The model under review builds one solid part; all positions refer to its coordinate system, in mm. A direction names the side the tool comes from. Coordinates: 2 decimals unless noted, no trailing zeros. Order: outer loops, then holes, each group sorted by start corner. A loop starts at its lowest first (then second) coordinate and runs counter-clockwise, first axis right, second up. Notation, with made-up numbers: (26.5, 46) -> (47.5, 46) arc R31 cw to (47.5, 72) -> close; hole circle Ø1 at (-31.5, 41). An arc over 180 degrees is marked (long way). Use one line per item in the form item = value.
from build123d import *

# Parameters (mm, degrees)
SKETCH_1_W           = 100
SKETCH_1_H           = 125
EXTRUDE_1_DEPTH      = 3
SKETCH_2_W           = 5
SKETCH_2_H           = 100
EXTRUDE_2_DEPTH      = 75
SKETCH_3_R           = 2.25
CUT_EXTRUDE_1_DEPTH  = 85
SKETCH_4_W           = 40
SKETCH_4_H           = 41.42
CUT_EXTRUDE_2_DEPTH  = 85
CHAMFER_1_SIZE       = 10
SKETCH_5_W           = 10
SKETCH_5_H           = 30
CUT_EXTRUDE_3_DEPTH  = 85
SKETCH_11_R          = 1.7
CUT_EXTRUDE_5_DEPTH  = 10
SKETCH_12_R          = 1.7
CUT_EXTRUDE_6_DEPTH  = 25
SKETCH_13_R          = 2.3
SKETCH_13_R_2        = 15
CUT_EXTRUDE_9_DEPTH  = 105
SKETCH_14_W          = 15
SKETCH_14_H          = 41.42
CUT_EXTRUDE_10_DEPTH = 83
SKETCH_15_W          = 38.97610678
SKETCH_15_H          = 41.42
CUT_EXTRUDE_11_DEPTH = 83
SKETCH_16_R          = 1.7
CUT_EXTRUDE_12_DEPTH = 83
SKETCH_17_R          = 2.15
CUT_EXTRUDE_13_DEPTH = 83
CHAMFER_2_SIZE       = 8


with BuildPart() as part:
    # 草图1 → 凸台-拉伸1 (new body)
    with BuildSketch(Plane(origin=(0, 0, 0), x_dir=(1, 0, 0), z_dir=(0, 1, 0))):
        Rectangle(SKETCH_1_W, SKETCH_1_H)
    extrude(amount=EXTRUDE_1_DEPTH)

    # 草图2 → 凸台-拉伸2 (add)
    with BuildSketch(Plane.XZ):
        with Locations((-34.5, 0)):
            Rectangle(SKETCH_2_W, SKETCH_2_H)
        with Locations((34.5, 0)):
            Rectangle(SKETCH_2_W, SKETCH_2_H)
    extrude(amount=EXTRUDE_2_DEPTH)

    # 草图3 → 切除-拉伸1 (cut)
    with BuildSketch(Plane.ZY.offset(37)):
        with Locations((-4.925, -12)):
            Circle(SKETCH_3_R)
        with Locations((4.925, -12)):
            Circle(SKETCH_3_R)
        with Locations((-4.925, -61.42)):
            Circle(SKETCH_3_R)
        with Locations((4.925, -61.42)):
            Circle(SKETCH_3_R)
        with Locations((14.775, -12)):
            Circle(SKETCH_3_R)
        with Locations((14.775, -61.42)):
            Circle(SKETCH_3_R)
        with Locations((-14.775, -61.42)):
            Circle(SKETCH_3_R)
        with Locations((-14.775, -12)):
            Circle(SKETCH_3_R)
    extrude(amount=-CUT_EXTRUDE_1_DEPTH, mode=Mode.SUBTRACT)

    # 草图4 → 切除-拉伸2 (cut)
    with BuildSketch(Plane.ZY.offset(37)):
        with Locations((0, -36.71)):
            Rectangle(SKETCH_4_W, SKETCH_4_H)
    extrude(amount=-CUT_EXTRUDE_2_DEPTH, mode=Mode.SUBTRACT)

    # 倒角1
    chamfer_1_edges = [part.edges().sort_by_distance(p)[0] for p in [
        (-34.5, -75, 50),
        (-34.5, -75, -50),
        (34.5, -75, 50),
        (34.5, -75, -50),
    ]]
    chamfer(chamfer_1_edges, length=CHAMFER_1_SIZE)

    # 草图5 → 切除-拉伸3 (cut)
    with BuildSketch(Plane(origin=(0, 3, 0), x_dir=(1, 0, 0), z_dir=(0, 1, 0))):
        with Locations((-25, 0)):
            Rectangle(SKETCH_5_W, SKETCH_5_H)
        with Locations((25, 0)):
            Rectangle(SKETCH_5_W, SKETCH_5_H)
    extrude(amount=-CUT_EXTRUDE_3_DEPTH, mode=Mode.SUBTRACT)

    # 草图11 → 切除-拉伸5 (cut)
    with BuildSketch(Plane.XZ):
        with Locations(Location((-44, 50.5, 0), (0, 0, 270))):
            Circle(SKETCH_11_R)
        with Locations(Location((-44, 38.5, 0), (0, 0, 270))):
            Circle(SKETCH_11_R)
        with Locations(Location((-44, 26.5, 0), (0, 0, 270))):
            Circle(SKETCH_11_R)
        with Locations(Location((44, 26.5, 0), (0, 0, 270))):
            Circle(SKETCH_11_R)
        with Locations(Location((44, 38.5, 0), (0, 0, 270))):
            Circle(SKETCH_11_R)
        with Locations(Location((44, 50.5, 0), (0, 0, 270))):
            Circle(SKETCH_11_R)
        with Locations(Location((44, -50.5, 0), (0, 0, 270))):
            Circle(SKETCH_11_R)
        with Locations(Location((44, -38.5, 0), (0, 0, 270))):
            Circle(SKETCH_11_R)
        with Locations(Location((44, -26.5, 0), (0, 0, 270))):
            Circle(SKETCH_11_R)
        with Locations(Location((-44, -26.5, 0), (0, 0, 270))):
            Circle(SKETCH_11_R)
        with Locations(Location((-44, -38.5, 0), (0, 0, 270))):
            Circle(SKETCH_11_R)
        with Locations(Location((-44, -50.5, 0), (0, 0, 270))):
            Circle(SKETCH_11_R)
    extrude(amount=-CUT_EXTRUDE_5_DEPTH, mode=Mode.SUBTRACT)

    # 草图12 → 切除-拉伸6 (cut)
    with BuildSketch(Plane(origin=(0, 3, 0), x_dir=(1, 0, 0), z_dir=(0, 1, 0))):
        with Locations(Location((-27.75, 54.5, 0), (0, 0, 270))):
            Circle(SKETCH_12_R)
        with Locations(Location((-27.75, 35.7, 0), (0, 0, 270))):
            Circle(SKETCH_12_R)
        with Locations(Location((27.75, 35.7, 0), (0, 0, 90))):
            Circle(SKETCH_12_R)
        with Locations(Location((27.75, 54.5, 0), (0, 0, 90))):
            Circle(SKETCH_12_R)
        with Locations(Location((27.75, -54.5, 0), (0, 0, 270))):
            Circle(SKETCH_12_R)
        with Locations(Location((27.75, -35.7, 0), (0, 0, 270))):
            Circle(SKETCH_12_R)
        with Locations(Location((-27.75, -35.7, 0), (0, 0, 90))):
            Circle(SKETCH_12_R)
        with Locations(Location((-27.75, -54.5, 0), (0, 0, 90))):
            Circle(SKETCH_12_R)
    extrude(amount=-CUT_EXTRUDE_6_DEPTH, mode=Mode.SUBTRACT)

    # 草图13 → 切除-拉伸9 (cut)
    with BuildSketch(Plane.ZY.offset(37)):
        with Locations((46, -16)):
            Circle(SKETCH_13_R)
        with Locations((46, -51)):
            Circle(SKETCH_13_R)
        with Locations((46, -33.5)):
            Circle(SKETCH_13_R_2)
    extrude(amount=-CUT_EXTRUDE_9_DEPTH, mode=Mode.SUBTRACT)

    # 草图14 → 切除-拉伸10 (cut)
    with BuildSketch(Plane.ZY.offset(37)):
        with Locations((-27.5, -36.71)):
            Rectangle(SKETCH_14_W, SKETCH_14_H)
    extrude(amount=-CUT_EXTRUDE_10_DEPTH, mode=Mode.SUBTRACT)

    # 草图15 → 切除-拉伸11 (cut)
    with BuildSketch(Plane.ZY.offset(37)):
        with Locations((-35, -36.71)):
            Rectangle(SKETCH_15_W, SKETCH_15_H)
    extrude(amount=-CUT_EXTRUDE_11_DEPTH, mode=Mode.SUBTRACT)

    # 草图16 → 切除-拉伸12 (cut)
    with BuildSketch(Plane(origin=(0, 3, 0), x_dir=(1, 0, 0), z_dir=(0, 1, 0))):
        with Locations(Location((-12.5, 15, 0), (0, 0, 270))):
            Circle(SKETCH_16_R)
        with Locations(Location((12.5, 15, 0), (0, 0, 90))):
            Circle(SKETCH_16_R)
        with Locations(Location((12.5, -15, 0), (0, 0, 270))):
            Circle(SKETCH_16_R)
        with Locations(Location((-12.5, -15, 0), (0, 0, 90))):
            Circle(SKETCH_16_R)
    extrude(amount=-CUT_EXTRUDE_12_DEPTH, mode=Mode.SUBTRACT)

    # 草图17 → 切除-拉伸13 (cut)
    with BuildSketch(Plane.ZY.offset(37)):
        with Locations((-24.625, -12)):
            Circle(SKETCH_17_R)
        with Locations((-24.625, -61.42)):
            Circle(SKETCH_17_R)
        with Locations((-39.625, -12)):
            Circle(SKETCH_17_R)
        with Locations((-39.625, -61.42)):
            Circle(SKETCH_17_R)
    extrude(amount=-CUT_EXTRUDE_13_DEPTH, mode=Mode.SUBTRACT)

    # 倒角2
    chamfer_2_edges = [part.edges().sort_by_distance(p)[0] for p in [
        (34.5, -16, -50),
        (-34.5, -16, -50),
    ]]
    chamfer(chamfer_2_edges, length=CHAMFER_2_SIZE)


solid = part.part
Item 1: To check wall thickness, follow L1, parallel to Y at x = -32.5, z = 15; L2, parallel to Y at x = 35.5, z = -33; L3, parallel to X at y = 2, z = -50. State the ranges of each line that lie inside material, in increasing order. Write a range as from..to.
Results found:
L1 = -75..-63.66, -59.18..-57.42, -16..-14.24, -9.76..3
L2 = -75..-57.42, -16..3
L3 = -50..-45.62, -42.38..42.38, 45.62..50
Item 2: We need section C-C (x = -44). Write out the cut boundary in (y, z), plus the area to 3 significant figures.
Results found:
outline = (0, -62.5) -> (3, -62.5) -> (3, -52.2) -> (0, -52.2) -> close; (0, -48.8) -> (3, -48.8) -> (3, -40.2) -> (0, -40.2) -> close; (0, -36.8) -> (3, -36.8) -> (3, -28.2) -> (0, -28.2) -> close; (0, -24.8) -> (3, -24.8) -> (3, 24.8) -> (0, 24.8) -> close; (0, 28.2) -> (3, 28.2) -> (3, 36.8) -> (0, 36.8) -> close; (0, 40.2) -> (3, 40.2) -> (3, 48.8) -> (0, 48.8) -> close; (0, 52.2) -> (3, 52.2) -> (3, 62.5) -> (0, 62.5) -> close
area = 314 mm²
Item 3: We need section A-A (z = 26.5). Write out the cut boundary in (x, y).
Results found:
outline = (-50, 0) -> (-45.7, 0) -> (-45.7, 3) -> (-50, 3) -> close; (-42.3, 0) -> (-37, 0) -> (-37, -75) -> (-32, -75) -> (-32, 0) -> (32, 0) -> (32, -75) -> (37, -75) -> (37, 0) -> (42.3, 0) -> (42.3, 3) -> (-42.3, 3) -> close; (45.7, 0) -> (50, 0) -> (50, 3) -> (45.7, 3) -> close
Item 4: Draft analysis for pull direction Z (two halves, no side actions). For faces 6 (the face through (-35, -9, 50)), 7 (the face through (-35, -12, -46)), 8 (the face through (42.34, 1.48, 38.87)), state which applies: released by +Z, released by -Z, zero draft, split by the parting line, or undercut.
Results found:
face_6 = released by +Z
face_7 = released by -Z
face_8 = undercut
Item 5: We need section D-D (z = 10.5). Write out the cut boundary in (x, y), plus the area to 3 significant figures.
Results found:
outline = (-50, 0) -> (-37, 0) -> (-37, -16) -> (-32, -16) -> (-32, 0) -> (-30, 0) -> (-30, 3) -> (-50, 3) -> close; (-37, -75) -> (-32, -75) -> (-32, -57.42) -> (-37, -57.42) -> close; (-20, 0) -> (20, 0) -> (20, 3) -> (-20, 3) -> close; (30, 0) -> (32, 0) -> (32, -16) -> (37, -16) -> (37, 0) -> (50, 0) -> (50, 3) -> (30, 3) -> close; (32, -75) -> (37, -75) -> (37, -57.42) -> (32, -57.42) -> close
area = 576 mm²
Item 6: We need section B-B (y = -3). Write out the cut boundary in (x, z), plus the area to 3 significant figures.
Results found:
outline = (-37, -50) -> (-32, -50) -> (-32, 50) -> (-37, 50) -> close; (32, -50) -> (37, -50) -> (37, 50) -> (32, 50) -> close
area = 1,000 mm²
Item 7: Clearance check with flat-ended pins moving along their axes: pin 1 (4.5 mm diameter, centred on x = -44, z = -26.5, fed in from +Y); pin 2 (2.5 mm diameter, centred on x = -35.5, y = -5.5, fed in from -Z); pin 3 (7 mm diameter, centred on y = -12, z = -39.625, fed in from -X); pin 4 (10 mm diameter, centred on y = -49, z = 41, fed in from +X). State where each tip first meets the part, or that it passes through.
Results found:
pin_1 = 3
pin_2 = -50
pin_3 = -37
pin_4 = 37
Item 8: Tool access review of faces 1 (the face through (-34.535, -11.354, -37.574)), 2 (the face through (34, -37, 20)), 3 (the face through (-35, -75, 1)), 4 (the face through (-25, 2, 15)), 5 (the face through (34, -56, 50)): name each direction out of +Z, -Z, +X, -X, +Y, -Y from which nothing blocks a thin tool from reaching the whole face with its end or side.
Results found:
face_1 = +X, -X
face_2 = -Z, +X, -X
face_3 = +Z, -Z, +X, -X, -Y
face_4 = +Y, -Y
face_5 = +Z, +X, -X, -Y
